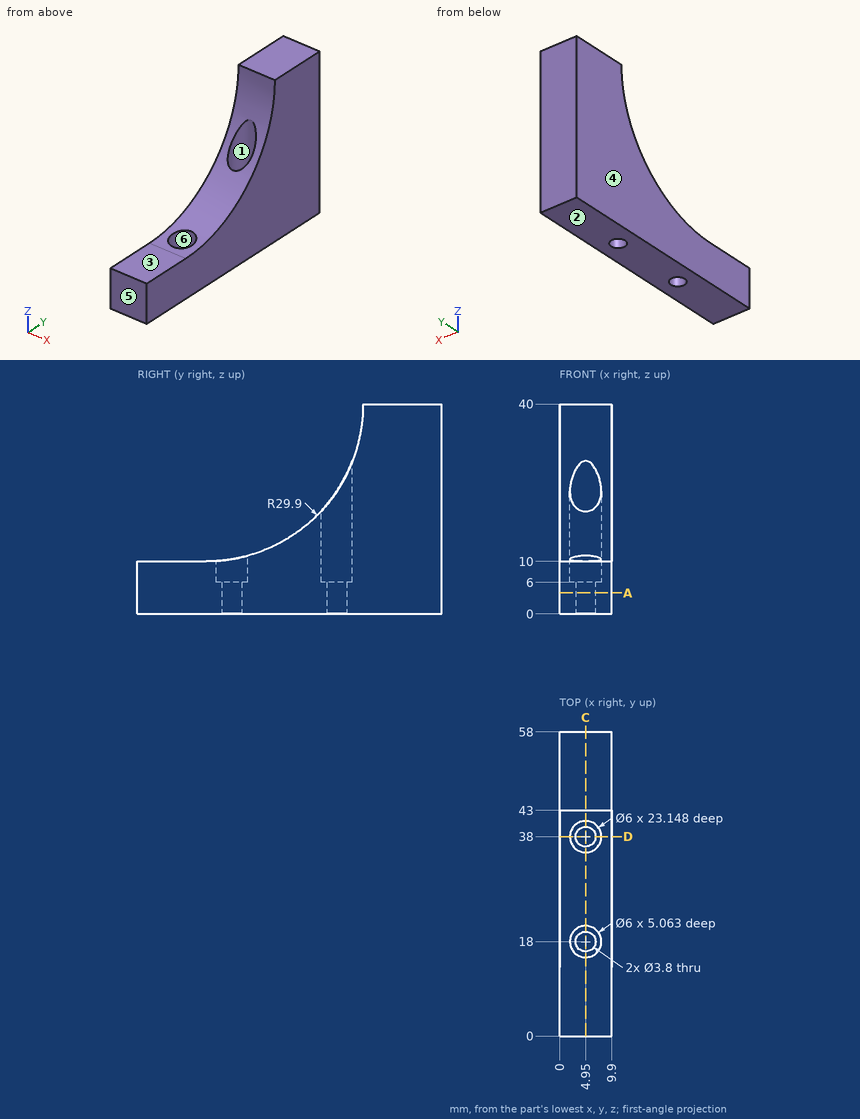
Part print with two shaded views. Sizes in mm from the minimum x, y, z corner. A direction names the side the tool comes from. Round coordinates to 2 decimals unless told otherwise and drop trailing zeros. Loops run counter-clockwise (first coordinate to the right, second up) from the corner with the lowest first, then second, coordinate; pieces in that order, holes last. Notation, with made-up numbers: (60.25, -26) - (96.25, -26) arc R27 ccw to (96.25, 3) - close; hole circle Ø4 at (-22, 39). An arc over 180 degrees is marked (long way). Answer as a JSON object with one key per item and string values.
Item 1: Band-saw the part on D-D on y = 38. List the corners of the cut face in (x, z).
Output:
{"outline": "(0, 0) - (3.05, 0) - (3.05, 6) - (1.95, 6) - (1.95, 23.35) - (0, 23.35) - close; (6.85, 0) - (9.9, 0) - (9.9, 23.35) - (7.95, 23.35) - (7.95, 6) - (6.85, 6) - close"}
Item 2: Pull direction Y, two halves, no side cores. Call the marked faces 4, 5 and 6: pulls with the +Y half, pulls with the -Y half, needs draft (parallel to the pull), parting line crosses it, or undercut.
Output:
{"face 4": "needs draft", "face 5": "pulls with the -Y half", "face 6": "undercut"}
Item 3: Band-saw the part on C-C on x = 4.95. List the corners of the cut face in (y, z).
Output:
{"outline": "(0, 0) - (16.1, 0) - (16.1, 6) - (15, 6) - (15, 10.06) arc R29.9 cw to (13.1, 10) - (0, 10) - close; (19.9, 0) - (36.1, 0) - (36.1, 6) - (35, 6) - (35, 19.54) arc R29.9 cw to (21, 11.06) - (21, 6) - (19.9, 6) - close; (39.9, 0) - (58, 0) - (58, 40) - (43, 40) - (43, 39.9) arc R29.9 cw to (41, 29.15) - (41, 6) - (39.9, 6) - close"}
Item 4: Band-saw the part on A-A on z = 4. List the corners of the cut face in (x, y).
Output:
{"outline": "(0, 0) - (9.9, 0) - (9.9, 58) - (0, 58) - close; hole circle Ø3.8 at (4.95, 18); hole circle Ø3.8 at (4.95, 38)"}
Item 5: Pin check, flat tips, straight feed: pin 1 (3 mm diameter, centred on x = 4.95, y = 38, fed in from -Z); pin 2 (5 mm diameter, centred on x = 5, y = 9.5, fed in from +Z); pin 3 (2 mm diameter, centred on x = 7.5, z = 20.5, fed in from -Y); pin 4 (3 mm diameter, centred on x = 4, y = 18, fed in from +Z). Stop position of each tip, or through.
Output:
{"pin 1": "through", "pin 2": "z = 10", "pin 3": "y = 34.96", "pin 4": "z = 6"}
Item 6: Wall check: L1, parallel to Y at x = 4.95, z = 4.15; L2, parallel to Y at x = 4.95, z = 7.6; L3, parallel to X at y = 38, z = 23. Give the ranges that are in metal, low to high.
Output:
{"L1": "0 to 16.1, 19.9 to 36.1, 39.9 to 58", "L2": "0 to 15, 21 to 35, 41 to 58", "L3": "0 to 1.95, 7.95 to 9.9"}
Item 7: Tool access for the marked faces 1, 2 and 3: list every direction of +Z, -Z, +X, -X, +Y, -Y with a clear straight run to the whole face (end or side of a thin tool).
Output:
{"face 1": "+Z", "face 2": "-Z, +X, -X, +Y, -Y", "face 3": "+Z, +X, -X, -Y"}
